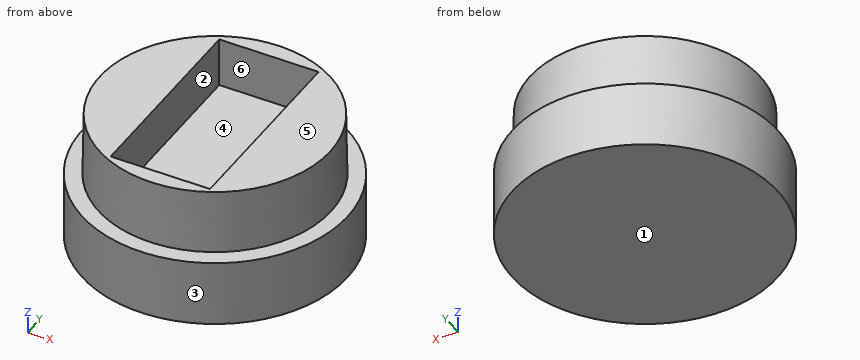
Autodesk Inventor part; units mm, degrees
ref_plane "YZ Plane" through (0, 0, 0) normal (1, 0, 0) x (0, 1, 0)
ref_plane "XZ Plane" through (0, 0, 0) normal (0, 1, 0) x (-1, 0, 0)
ref_plane "XY Plane" through (0, 0, 0) normal (0, 0, 1) x (1, 0, 0)
sketch "Sketch1" plane through (0, 0, 0) normal (0, 0, 1) x (1, 0, 0)
  circle A0 centre (0, 0) radius 35.25
  circle A1 centre (0, 0) radius 40
  dimension "d0" = 70.5
  dimension "d4" = 80
extrude "Extrusion1" add sketch "Sketch1" along normal blind 29.5 contours A0
draft "FaceDraft1" angle 1 pull direction (0, 0, 1) faces at (35.144, -2.7316, 19.6667) fixed edges at (-35.25, 0, 0)
extrude "Extrusion2" add sketch "Sketch1" along normal mid plane 20 contours A0 | A1
sketch "Skizze2" plane through (0, 0, 29.5) normal (0, 0, 1) x (1, 0, 0)
  circle A0 centre (0, 0) radius 34.7351
  line L0 (-21.0374, 27.6397) -> (-15.0374, 27.6397)
  line L1 (-15.0374, 27.6397) -> (-15.0374, 26.6397)
  line L2 (-15.0374, 26.6397) -> (-21.0374, 26.6397)
  line L3 (-21.0374, 26.6397) -> (-21.0374, 27.6397)
  line L4 (-15.0374, 26.6397) -> (14.9626, 26.6397)
  line L5 (14.9626, 26.6397) -> (14.9626, -29.8603)
  line L6 (14.9626, -29.8603) -> (-15.0374, -29.8603)
  line L7 (-15.0374, -29.8603) -> (-15.0374, 26.6397)
  line L8 (-15.0374, 26.6397) -> (14.9626, 26.6397)
  line L9 (14.9626, 26.6397) -> (14.9626, 29.6397)
  line L10 (14.9626, 29.6397) -> (-15.0374, 29.6397)
  line L11 (-15.0374, 29.6397) -> (-15.0374, 26.6397)
  dimension "d7" = 6
  dimension "d8" = 1
  dimension "d9" = 30
  dimension "d10" = 56.5
  dimension "d11" = 3
extrude "Extrusion3" cut sketch "Skizze2" against normal blind 15 contours L11 L10 L9 L4 L1 | L4 L5 L6 L7
properties part number "stopfen-front" material "yellow foam"
For this review, take the finished solid that the model builds, in its own axes (mm). Face numbers are marked on the shaded views. A direction names the side the tool comes from. Coordinates: 2 decimals unless noted, no trailing zeros. Loops run counter-clockwise (first coordinate to the right, second up) from the corner with the lowest first, then second, coordinate; pieces in that order, holes last.
1. Mouldability with a two-part tool opening along Y and no side actions: class the marked faces 1, 2, 3 and 4 as +Y half, -Y half, draft (parallel to the pull), parting line (faces both ways), or undercut.
2. For line 1 (Z direction, x = 32.5, y = 19); line 2 (Y direction, x = 0, z = 8); line 3 (Y direction, x = 1, z = 23), list the stretches that pass through material, from the lowest coordinate up.
3. Insertion check: P1, Ø4, axis at x = -19.5, z = 15.5, coming from the -Y side; P2, Ø8, axis at y = 25, z = 7, coming from the -X side; P3, Ø9, axis at x = -1, y = -3.5, coming from the +Z side. Each pin has a flat end and moves straight along its axis. Give the tip position at first contact, or say it passes through.
4. Add section A-A, the plane z = -3.5. Give the boundary of the cut face in (x, y), then the cut area to 3 significant figures.
5. For the marked faces 5 and 6, list the 3-axis set-ups (+Z, -Z, +X, -X, +Y, -Y) from which the entire face can be reached by the end or side of a thin tool; tool diameter is ignored.
Result:
1. face 1: draft
1. face 2: undercut
1. face 3: parting line
1. face 4: undercut
2. line 1: z = -10 to 10
2. line 2: y = -40 to 40
2. line 3: y = -34.83 to -29.86, 29.64 to 34.83
3. P1: stops at y = -30.29
3. P2: stops at x = -34.04
3. P3: stops at z = 14.5
4. outline: circle Ø80 at (0, 0)
4. area: 5,030 mm2
5. face 5: +Z, +X, -X, +Y, -Y
5. face 6: +Z
